```python
from build123d import *

# Parameters (mm, degrees)
SKETCH1_W           = 203.2
SKETCH1_H           = 152.4
BOSS_EXTRUDE1_DEPTH = 3.175
SKETCH3_R           = 3.2512
CUT_EXTRUDE4_DEPTH  = 5.08
SKETCH2_R           = 25.4762
SKETCH2_R_2         = 14.2875
SKETCH2_R_3         = 9.525
SKETCH2_R_4         = 2.54
SKETCH2_R_5         = 9.5504
CUT_EXTRUDE5_DEPTH  = 50.8


with BuildPart() as part:
    # Sketch1 → Boss-Extrude1 (new body)
    with BuildSketch(Plane(origin=(0, 0, 0), x_dir=(1, 0, 0), z_dir=(0, 1, 0))):
        with Locations((101.6, 76.2)):
            Rectangle(SKETCH1_W, SKETCH1_H)
    extrude(amount=BOSS_EXTRUDE1_DEPTH)

    # Sketch3 → Cut-Extrude4 (cut)
    with BuildSketch(Plane(origin=(0, 3.175, 0), x_dir=(1, 0, 0), z_dir=(0, 1, 0))):
        with Locations(Location((12.7, 12.7, 0), (0, 0, 270))):  # turned: the seam where the file's is
            Circle(SKETCH3_R)
        with Locations(Location((38.1, 12.7, 0), (0, 0, 270))):  # turned: the seam where the file's is
            Circle(SKETCH3_R)
        with Locations(Location((63.5, 12.7, 0), (0, 0, 270))):  # turned: the seam where the file's is
            Circle(SKETCH3_R)
        with Locations(Location((88.9, 12.7, 0), (0, 0, 270))):  # turned: the seam where the file's is
            Circle(SKETCH3_R)
        with Locations(Location((114.3, 12.7, 0), (0, 0, 270))):  # turned: the seam where the file's is
            Circle(SKETCH3_R)
        with Locations(Location((139.7, 12.7, 0), (0, 0, 270))):  # turned: the seam where the file's is
            Circle(SKETCH3_R)
        with Locations(Location((165.1, 12.7, 0), (0, 0, 270))):  # turned: the seam where the file's is
            Circle(SKETCH3_R)
        with Locations(Location((190.5, 12.7, 0), (0, 0, 270))):  # turned: the seam where the file's is
            Circle(SKETCH3_R)
        with Locations(Location((190.5, 114.3, 0), (0, 0, 270))):  # turned: the seam where the file's is
            Circle(SKETCH3_R)
        with Locations(Location((190.5, 139.7, 0), (0, 0, 270))):  # turned: the seam where the file's is
            Circle(SKETCH3_R)
        with Locations(Location((12.7, 38.1, 0), (0, 0, 270))):  # turned: the seam where the file's is
            Circle(SKETCH3_R)
        with Locations(Location((12.7, 63.5, 0), (0, 0, 270))):  # turned: the seam where the file's is
            Circle(SKETCH3_R)
        with Locations(Location((12.7, 88.9, 0), (0, 0, 270))):  # turned: the seam where the file's is
            Circle(SKETCH3_R)
        with Locations(Location((12.7, 114.3, 0), (0, 0, 270))):  # turned: the seam where the file's is
            Circle(SKETCH3_R)
        with Locations(Location((12.7, 139.7, 0), (0, 0, 270))):  # turned: the seam where the file's is
            Circle(SKETCH3_R)
        with Locations(Location((38.1, 139.7, 0), (0, 0, 270))):  # turned: the seam where the file's is
            Circle(SKETCH3_R)
        with Locations(Location((63.5, 139.7, 0), (0, 0, 270))):  # turned: the seam where the file's is
            Circle(SKETCH3_R)
        with Locations(Location((88.9, 139.7, 0), (0, 0, 270))):  # turned: the seam where the file's is
            Circle(SKETCH3_R)
        with Locations(Location((114.3, 139.7, 0), (0, 0, 270))):  # turned: the seam where the file's is
            Circle(SKETCH3_R)
    extrude(amount=-CUT_EXTRUDE4_DEPTH, mode=Mode.SUBTRACT)

    # Sketch2 → Cut-Extrude5 (cut)
    with BuildSketch(Plane(origin=(0, 3.175, 0), x_dir=(1, 0, 0), z_dir=(0, 1, 0))):
        with Locations(Location((82.55, 82.55, 0), (0, 0, 270))):  # turned: the seam where the file's is
            Circle(SKETCH2_R)
        with Locations(Location((131.7498, 53.34, 0), (0, 0, 270))):  # turned: the seam where the file's is
            Circle(SKETCH2_R_2)
        with Locations(Location((167.4622, 59.69, 0), (0, 0, 270))):  # turned: the seam where the file's is
            Circle(SKETCH2_R_3)
        with Locations(Location((167.4622, 34.29, 0), (0, 0, 270))):  # turned: the seam where the file's is
            Circle(SKETCH2_R_4)
        with Locations(Location((167.4622, 85.09, 0), (0, 0, 270))):  # turned: the seam where the file's is
            Circle(SKETCH2_R_4)
        with Locations(Location((125.0696, 110.49, 0), (0, 0, 270))):  # turned: the seam where the file's is
            Circle(SKETCH2_R_2)
        with Locations(Location((161.8742, 120.65, 0), (0, 0, 270))):  # turned: the seam where the file's is
            Circle(SKETCH2_R_5)
        with Locations(Location((179.832, 102.6922, 0), (0, 0, 270))):  # turned: the seam where the file's is
            Circle(SKETCH2_R_4)
        with Locations(Location((143.9164, 138.6078, 0), (0, 0, 270))):  # turned: the seam where the file's is
            Circle(SKETCH2_R_4)
    extrude(amount=-CUT_EXTRUDE5_DEPTH, mode=Mode.SUBTRACT)


solid = part.part
```
Verification items for the finished model (mm, model axes). Coordinates: 2 decimals unless noted, no trailing zeros. Loops run counter-clockwise (first coordinate to the right, second up) from the corner with the lowest first, then second, coordinate; pieces in that order, holes last. Notation, with made-up numbers: (74, -14.5) -> (97, -14.5) arc R14 ccw to (97, 0.5) -> close; hole circle Ø3 at (24, 9). An arc over 180 degrees is marked (long way). Answer in a Markdown table with one row per item.
1) Section check B-B (z = -114.3). Record the cut outline in (x, y) (3 decimals), and give its area (3 significant figures).
The answers:
| item | result |
|---|---|
| outline | (0, 0) -> (9.449, 0) -> (9.449, 3.175) -> (0, 3.175) -> close; (15.951, 0) -> (111.299, 0) -> (111.299, 3.175) -> (15.951, 3.175) -> close; (138.84, 0) -> (154.741, 0) -> (154.741, 3.175) -> (138.84, 3.175) -> close; (169.008, 0) -> (187.249, 0) -> (187.249, 3.175) -> (169.008, 3.175) -> close; (193.751, 0) -> (203.2, 0) -> (203.2, 3.175) -> (193.751, 3.175) -> close |
| area | 471 mm2 |
2) Scan lines: line 1 along X through (y, z) = (3, -38); line 2 along Z through (x, y) = (63, 0.6); line 3 along Z through (x, y) = (130, 2.1). Record each from-to range of solid material in increasing order. Write a range as from..to.
The answers:
| item | result |
|---|---|
| line 1 | x = 0..9.45, 15.95..203.2 |
| line 2 | z = -152.4..-142.91, -136.49..-98.89, -66.21..-15.91, -9.49..0 |
| line 3 | z = -152.4..-123.9, -97.08..-67.52, -39.16..0 |
3) Draft check along Z on faces 1 (the face through (161.926, 1.61, -13.405)), 2 (the face through (100, 0, -60)). Enter one of: released by +Z, released by -Z, zero draft, split by the parting line, or undercut.
The answers:
| item | result |
|---|---|
| face 1 | undercut |
| face 2 | zero draft |
4) Section check C-C (y = 2.6). Give the number of separate pieces and of enclosed holes in the cut face, and give its area (3 significant figures).
The answers:
| item | result |
|---|---|
| separate pieces | 1 |
| enclosed holes | 28 |
| area | 26,400 mm2 |
5) Depth check by flat-ended pin: P1, Ø6, axis at x = 88.9, z = -139.7, coming from the -Y side. Enter the tip coordinate at first touch or a pass-through.
The answers:
| item | result |
|---|---|
| P1 | passes through |
6) Section check D-D (x = 114.3). Record the cut outline in (y, z) (3 decimals), and give its area (3 significant figures).
The answers:
| item | result |
|---|---|
| outline | (0, -152.4) -> (3.175, -152.4) -> (3.175, -142.951) -> (0, -142.951) -> close; (0, -136.449) -> (3.175, -136.449) -> (3.175, -119.879) -> (0, -119.879) -> close; (0, -101.101) -> (3.175, -101.101) -> (3.175, -15.951) -> (0, -15.951) -> close; (0, -9.449) -> (3.175, -9.449) -> (3.175, 0) -> (0, 0) -> close |
| area | 383 mm2 |
7) Section check A-A (x = 82.55). Record the cut outline in (y, z) (3 decimals), and give its area (3 significant figures).
The answers:
| item | result |
|---|---|
| outline | (0, -152.4) -> (3.175, -152.4) -> (3.175, -108.026) -> (0, -108.026) -> close; (0, -57.074) -> (3.175, -57.074) -> (3.175, 0) -> (0, 0) -> close |
| area | 322 mm2 |
